```python
from build123d import *

# Parameters (mm, degrees)
SKETCH1_R           = 5
BOSS_EXTRUDE1_DEPTH = 102.9
SKETCH2_W           = 28.867513459
SKETCH2_H           = 96.9
CUT_EXTRUDE1_DEPTH  = 217
BOSS_EXTRUDE2_DEPTH = 5


with BuildPart() as part:
    # Sketch1 → Boss-Extrude1 (new body)
    with BuildSketch(Plane(origin=(0, 0, 0), x_dir=(1, 0, 0), z_dir=(0, 1, 0))):
        with BuildLine():
            Line((-28.867513459, -84.364700653), (0, -84.364700653))
            Line((0, -84.364700653), (0, -100))
            ThreePointArc((0, -100), (-14.43375673, -114.43375673), (-28.867513459, -100))
            Line((-28.867513459, -100), (-28.867513459, -84.364700653))
        make_face()
        with Locations(Location((-14.43375673, -100, 0), (0, 0, 270))):
            Circle(SKETCH1_R, mode=Mode.SUBTRACT)
    extrude(amount=BOSS_EXTRUDE1_DEPTH)

    # Sketch2 → Cut-Extrude1 (cut)
    with BuildSketch(Plane.XY):
        with Locations((-14.43375673, 51.45)):
            Rectangle(SKETCH2_W, SKETCH2_H)
    extrude(amount=CUT_EXTRUDE1_DEPTH, mode=Mode.SUBTRACT)


with BuildPart() as cut_extrude1_piece_1:
    # of the separate pieces the step leaves, piece 1, a body of its own (cut_extrude1_pieces)
    add(part.part.solids().sort_by_distance((-28.867513459, 0, 100))[0])



with BuildPart() as cut_extrude1_piece_2:
    # of the separate pieces the step leaves, piece 2, a body of its own (cut_extrude1_pieces)
    add(part.part.solids().sort_by_distance((-28.867513459, 99.9, 84.364700653))[0])


with BuildPart() as cut_extrude1_piece_1_1:
    add(cut_extrude1_piece_1.part)

    add(cut_extrude1_piece_2.part)  # Boss-Extrude2 merges Cut-Extrude1 piece 2
    # Sketch5 → Boss-Extrude2 (add)
    with BuildSketch(Plane(origin=(0, 0, 84.364700653), x_dir=(-1, 0, 0), z_dir=(0, 0, -1))):
        with BuildLine():
            Line((-10, 112.9), (38.867513459, 112.9))
            ThreePointArc((38.867513459, 112.9), (45.938581271, 109.971067812), (48.867513459, 102.9))
            Line((48.867513459, 102.9), (48.867513459, 0))
            ThreePointArc((48.867513459, 0), (45.938581271, -7.071067812), (38.867513459, -10))
            Line((38.867513459, -10), (-10, -10))
            ThreePointArc((-10, -10), (-17.071067812, -7.071067812), (-20, 0))
            Line((-20, 0), (-20, 102.9))
            ThreePointArc((-20, 102.9), (-17.071067812, 109.971067812), (-10, 112.9))
        make_face()
    extrude(amount=BOSS_EXTRUDE2_DEPTH)


solid = cut_extrude1_piece_1_1.part
```
Input: part model. Units: mm. Frame: model coordinates. A direction names the side the tool comes from. Round coordinates to 2 decimals unless told otherwise and drop trailing zeros. Loops run counter-clockwise (first coordinate to the right, second up) from the corner with the lowest first, then second, coordinate; pieces in that order, holes last. Notation, with made-up numbers: (26, 53.25) -> (30, 53.25) arc R4 ccw to (30, 57.25) -> close; hole circle Ø2 at (37.5, 18.25). An arc over 180 degrees is marked (long way). Write each question's results on one line, items separated by ' | '.
1. Ray query, line 1 (X direction, y = 101, z = 100); line 2 (Y direction, x = -18.5, z = 93); line 3 (Z direction, x = -18.5, y = 64). Return the intervals inside material, ascending. Write a range as from..to.
Geometry results:
line 1: -28.87..-19.43, -9.43..0 | line 2: 0..3, 99.9..102.9 | line 3: 79.36..84.36
2. Section A-A (z = 88.5). Return loops of the section in (x, y).
Geometry results:
outline: (-28.87, 0) -> (0, 0) -> (0, 3) -> (-28.87, 3) -> close; (-28.87, 99.9) -> (0, 99.9) -> (0, 102.9) -> (-28.87, 102.9) -> close
3. First-contact query: P1, Ø16, axis at x = -14.43, z = 100, coming from the +Y side; P2, Ø8.5, axis at x = -19.5, z = 96.5, coming from the -Y side; P3, Ø2.5, axis at y = 1.5, z = 95, coming from the +X side; P4, Ø1.5, axis at y = 91, z = 87, coming from the +X side. Flat tips, straight axial feed; report the tip coordinate or a pass-through.
Geometry results:
P1: y = 102.9 | P2: y = 0 | P3: x = 0 | P4: through
4. Mould query, pull axis Z, two halves, no side actions, for faces 6 (the face through (-16.35, 101.38, 104.62)), 7 (the face through (-11, 99.9, 96)), 8 (the face through (-15, 52, 79.365)). Classes: +Z half, -Z half, draft (parallel to the pull), parting line (faces both ways), or undercut.
Geometry results:
face 6: undercut | face 7: draft | face 8: -Z half
5. Section D-D (z = 111). Return loops of the section in (x, y), and give its area (3 significant figures).
Geometry results:
outline: (-23.78, 0) -> (-5.09, 0) -> (-5.09, 3) -> (-23.78, 3) -> close; (-23.78, 99.9) -> (-5.09, 99.9) -> (-5.09, 102.9) -> (-23.78, 102.9) -> close | area: 112 mm2
6. Section B-B (y = 1.5). Return loops of the section in (x, z).
Geometry results:
outline: (-48.87, 79.36) -> (20, 79.36) -> (20, 84.36) -> (0, 84.36) -> (0, 100) arc R14.43 ccw to (-28.87, 100) -> (-28.87, 84.36) -> (-48.87, 84.36) -> close; hole circle Ø10 at (-14.43, 100)
7. Set-up query: faces 1 (the face through (-11, 3, 96)), 2 (the face through (-15, -10, 82)), 3 (the face through (-28.868, 101, 92)), 4 (the face through (-11, 0, 96)), 5 (the face through (0, 1, 92)). Return all of +Z, -Z, +X, -X, +Y, -Y with unobstructed straight access to the full face (end or side cutting, diameter ignored); none if empty.
Geometry results:
face 1: +Z, +X, -X | face 2: +Z, -Z, +X, -X, -Y | face 3: +Z, -X, +Y, -Y | face 4: +Z, +X, -X, -Y | face 5: +Z, +X, +Y, -Y
8. Section C-C (x = 5.5). Return loops of the section in (y, z).
Geometry results:
outline: (-10, 79.36) -> (112.9, 79.36) -> (112.9, 84.36) -> (-10, 84.36) -> close
